Model file for the job. Use its own axes, mm. A direction names the side the tool comes from. Round coordinates to 2 decimals unless told otherwise and drop trailing zeros. Loops run counter-clockwise (first coordinate to the right, second up) from the corner with the lowest first, then second, coordinate; pieces in that order, holes last. Notation, with made-up numbers: M -6,20.25 L 49,20.25 A18 cw 49,53.25 Z; hole C 5.5,87 d11. An arc over 180 degrees is marked long. Use a Markdown table: item, result. Add a question column.
Item 1: Wall check: L1, parallel to Y at x = 6, z = 20; L2, parallel to Y at x = 11.25, z = 20; L3, parallel to Z at x = 28, y = 31.5. Give the ranges that are in metal, low to high. Write a range as from..to.
Item 2: Tool access for faces 4 (the flat face through (10, -27, 20)), 5 (the cylindrical face through (30.24, 22.3, -2.17)), 6 (the cylindrical face through (33.283, 29.649, 15.504)): list every direction of +Z, -Z, +X, -X, +Y, -Y with a clear straight run to the whole face (end or side of a thin tool).
Item 3: Saw through at B-B on z = -4. Write the cut outline in (x, y), then the cut area to 3 significant figures.
Item 4: Saw through at D-D on z = -20. Write the cut outline in (x, y).
Item 5: Saw through at C-C on y = 8. Write the cut outline in (x, z).
Item 6: Two-plate mould, pull along Z, no slides. Class faces 1 (the cylindrical face through (10.983, -25.348, -20.106)), 2 (the cylindrical face through (59.994, 24.323, 0.715)), 3 (the flat face through (3, -40, -1)): +Z half, -Z half, draft (parallel to the pull), parting line (faces both ways), or undercut.
Item 7: Saw through at A-A on x = 40. Write the cut outline in (y, z), then the cut area to 3 significant figures.
Item 8: Pin check, flat tips, straight feed: P1, Ø3, axis at y = -30, z = -19.5, coming from the -X side; P2, Ø8, axis at x = 46.5, y = 20, coming from the -Z side; P3, Ø7, axis at y = -29.85, z = -20, coming from the +X side; P4, Ø8, axis at y = -8, z = 26.5, coming from the +X side. Stop position of each tip, or through.
```python
from build123d import *

# Parameters (mm, degrees)
SKETCH2_R           = 10
BOSS_EXTRUDE1_DEPTH = 40
CUT_EXTRUDE1_DEPTH  = 40
SKETCH4_R           = 2.5
CUT_EXTRUDE2_DEPTH  = 80
SKETCH5_R           = 4.5
CUT_EXTRUDE3_DEPTH  = 80


with BuildPart() as part:
    # Sketch2 → Boss-Extrude1 (new, symmetric)
    with BuildSketch(Plane(origin=(0, 0, 0), x_dir=(1, 0, 0), z_dir=(0, 1, 0))):
        with BuildLine():
            Line((0, 40), (0, -40))
            Line((0, -40), (34.939220954, -40))
            ThreePointArc((34.939220954, -40), (60, -0.01901654), (35, 40))
            Line((35, 40), (0, 40))
        make_face()
        with Locations(Location((40, 0, 0), (0, 0, 270))):
            Circle(SKETCH2_R, mode=Mode.SUBTRACT)
    extrude(amount=BOSS_EXTRUDE1_DEPTH, both=True)

    # Sketch3 → Cut-Extrude1 (cut, symmetric)
    with BuildSketch(Plane.XY):
        with BuildLine():
            Line((60.000012836, 9.630791914), (60.000012836, -40))
            Line((60.000012836, -40), (6.370793002, -40))
            ThreePointArc((6.370793002, -40), (26.384718506, -7.836033018), (60.000012836, 9.630791914))
        make_face()
    extrude(amount=CUT_EXTRUDE1_DEPTH, both=True, mode=Mode.SUBTRACT)

    # Sketch4 → Cut-Extrude2 (cut)
    with BuildSketch(Plane(origin=(0, 0, 0), x_dir=(0, 0, -1), z_dir=(1, 0, 0))):
        with Locations(Location((-20, 29.846630116, 0), (0, 0, 180))):
            Circle(SKETCH4_R)
        with Locations(Location((20, 29.846630116, 0), (0, 0, 180))):
            Circle(SKETCH4_R)
        with Locations(Location((20, -29.846630116, 0), (0, 0, 180))):
            Circle(SKETCH4_R)
        with Locations(Location((-20, -29.846630116, 0), (0, 0, 180))):
            Circle(SKETCH4_R)
    extrude(amount=CUT_EXTRUDE2_DEPTH, mode=Mode.SUBTRACT)

    # Sketch5 → Cut-Extrude3 (cut)
    with BuildSketch(Plane(origin=(10, 0, 0), x_dir=(0, 0, -1), z_dir=(1, 0, 0))):
        with Locations(Location((20, 29.846630116, 0), (0, 0, 180))):
            Circle(SKETCH5_R)
        with Locations(Location((-20, 29.846630116, 0), (0, 0, 180))):
            Circle(SKETCH5_R)
        with Locations((20, -29.846630116)):
            Circle(SKETCH5_R)
        with Locations((-20, -29.846630116)):
            Circle(SKETCH5_R)
    extrude(amount=CUT_EXTRUDE3_DEPTH, mode=Mode.SUBTRACT)


solid = part.part
```
Entries:
| question | item | result |
|---|---|---|
| 1 | L1 | -40..-32.35, -27.35..27.35, 32.35..40 |
| 1 | L2 | -25.35..25.35, 34.35..40 |
| 1 | L3 | -40..-24.19, -15.81..15.81, 24.19..40 |
| 2 | face 4 | +X, -Y |
| 2 | face 5 | +Y, -Y |
| 2 | face 6 | +X |
| 3 | outline | M 0,-40 L 6.37,-40 A71.66 cw 30.83,-4.04 L 30.83,40 L 0,40 Z; M 49.17,6.39 A71.66 cw 59.82,9.59 L 59.82,40 L 49.17,40 Z |
| 3 | area | 2,270 mm2 |
| 4 | outline | M 0,-40 L 6.37,-40 A71.66 cw 9.13,-32.35 L 0,-32.35 Z; M 0,-27.35 L 10,-27.35 L 10,-25.35 L 12.57,-25.35 A71.66 cw 55.26,8.44 L 55.26,25.35 L 10,25.35 L 10,27.35 L 0,27.35 Z; M 0,32.35 L 10,32.35 L 10,34.35 L 55.26,34.35 L 55.26,40 L 0,40 Z |
| 5 | outline | M 0,-40 L 35,-40 A44.48 ccw 53.78,-22.69 L 53.78,22.66 A44.48 ccw 34.94,40 L 0,40 Z; hole C 40,0 d20 |
| 6 | face 1 | undercut |
| 6 | face 2 | parting line |
| 6 | face 3 | draft |
| 7 | outline | M 2.07,-37.15 L 40,-37.15 L 40,-10 L 2.07,-10 Z; M 2.07,10 L 40,10 L 40,37.12 L 2.07,37.12 Z; hole C 29.85,-20 d9; hole C 29.85,20 d9 |
| 7 | area | 1,930 mm2 |
| 8 | P1 | through |
| 8 | P2 | z = -35.38 |
| 8 | P3 | x = 10 |
| 8 | P4 | x = 30.89 |
